```python
from build123d import *

# Parameters (mm, degrees)
CROQUIS1_W              = 670
CROQUIS1_H              = 125
SALIENTE_EXTRUIR1_DEPTH = 22
CROQUIS2_W              = 11
CROQUIS2_H              = 22
CORTAR_EXTRUIR1_DEPTH   = 676.706056466


with BuildPart() as part:
    # Croquis1 → Saliente-Extruir1 (new body)
    with BuildSketch(Plane.XY):
        with Locations((200.670606996, 22.321428571)):
            Rectangle(CROQUIS1_W, CROQUIS1_H)
    extrude(amount=SALIENTE_EXTRUIR1_DEPTH)

    # Croquis2 → Cortar-Extruir1 (cut, through all)
    with BuildSketch(Plane.ZY.offset(134.329393004)):
        with Locations((16.5, -29.178571429)):
            Rectangle(CROQUIS2_W, CROQUIS2_H)
    extrude(amount=-CORTAR_EXTRUIR1_DEPTH, mode=Mode.SUBTRACT)


solid = part.part
```
Read the model definition and answer for the solid it produces. Units are mm, in the model's axes. A direction names the side the tool comes from. Give positions to 0.01 mm unless a question says otherwise; leave off trailing zeros. Order: outer loops, then holes, each group sorted by start corner. A loop starts at its lowest first (then second) coordinate and runs counter-clockwise, first axis right, second up.
(1) Given pin 1 (17.5 mm diameter, centred on x = 319.5, y = -27, fed in from +Z), flat-ended and moving along its own axis, determine where the tip first touches the part or whether it passes through.
(2) Straight lines are drawn through the part: L1, parallel to Y at x = 151, z = 13.25; L2, parallel to Z at x = 228, y = -28.5. For each, find the intervals that lie inside material, in ascending order.
(3) For a pull along Z with two mould halves and no side action, classify faces 3 (the flat face through (196, -18.179, 16)), 4 (the flat face through (196, 34, 22)), 5 (the flat face through (196, 23, 0)) as released by +Z, released by -Z, zero draft, split by the parting line, or undercut.
(4) Find section B-B (z = 15.5). Give the vertices of the cut face in (x, y), plus the area to 3 significant figures.
(5) Find section A-A (x = 246). Give the vertices of the cut face in (y, z), plus the area to 3 significant figures.
(6) For faces 1 (the flat face through (535.671, 21, 11)), 2 (the flat face through (196, -29, 11)), determine the directions among +Z, -Z, +X, -X, +Y, -Y from which every point of the face is accessible in a straight line to the end or side of a thin tool.
Result sheet:
1. pin 1: stops at z = 11
2. L1: y = -18.18 to 84.82
2. L2: z = 0 to 11
3. face 3: zero draft
3. face 4: released by +Z
3. face 5: released by -Z
4. outline: (-134.33, -18.18) - (535.67, -18.18) - (535.67, 84.82) - (-134.33, 84.82) - close
4. area: 69,000 mm2
5. outline: (-40.18, 0) - (84.82, 0) - (84.82, 22) - (-18.18, 22) - (-18.18, 11) - (-40.18, 11) - close
5. area: 2,510 mm2
6. face 1: +Z, -Z, +X, +Y, -Y
6. face 2: +Z, +X, -X, -Y
